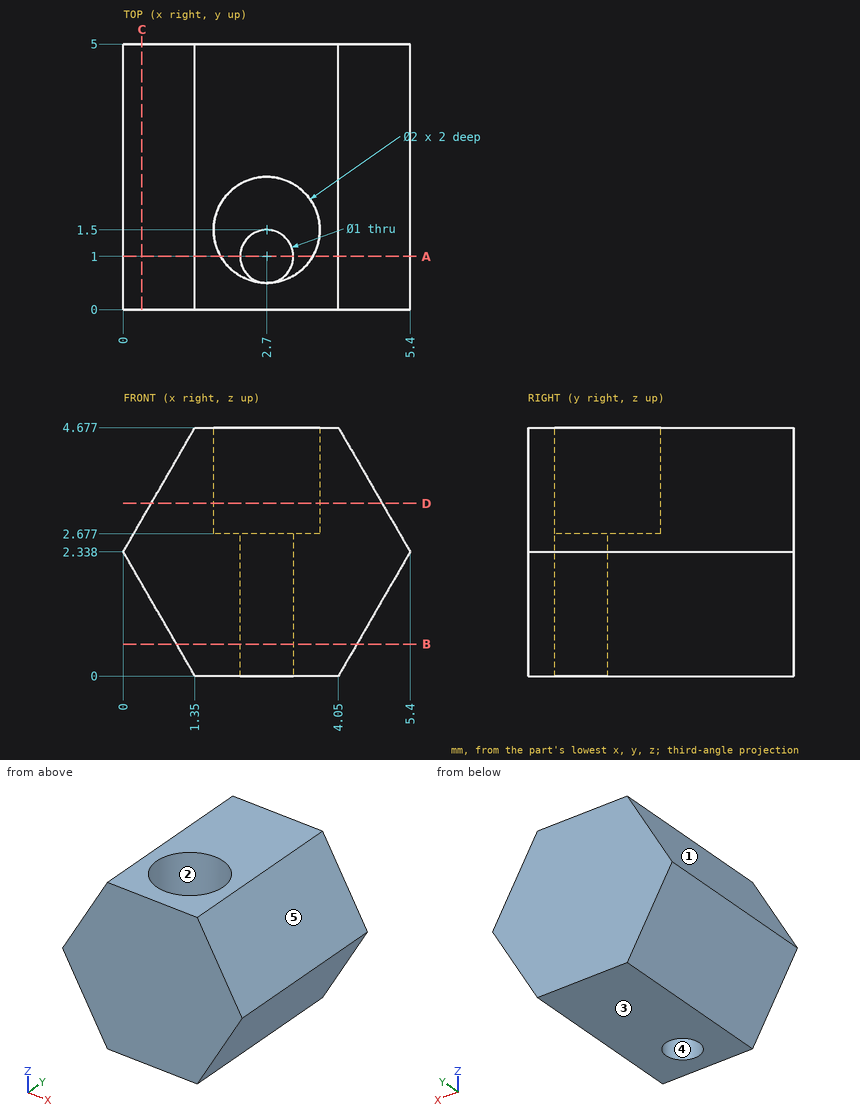
Geometry check sheet. Reference: drawing and pictorial views, mm from the part's lowest x, y, z. A direction names the side the tool comes from. Give positions to 0.01 mm unless a question says otherwise; leave off trailing zeros. Loops run counter-clockwise (first coordinate to the right, second up) from the corner with the lowest first, then second, coordinate; pieces in that order, holes last. Notation, with made-up numbers: M 15,33 L 20,33 A23 ccw 20,49 Z; hole C 69,47.25 d8. An arc over 180 degrees is marked long. Use a Markdown table: item, result. Add a question column.
Q1. Scan lines: line 1 along Y through (x, z) = (2.7, 2.05); line 2 along Y through (x, z) = (2.7, 3.25); line 3 along X through (y, z) = (1, 1.7). Record each from-to range of solid material in increasing order. Write a range as [from, to].
Q2. Go/stop test with flat-tipped pins: pin 1 (1 mm diameter, centred on y = 3, z = 1, fed in from +X) (1 decimal); pin 2 (1 mm diameter, centred on x = 5, y = 2.5, fed in from -Z); pin 3 (1.6 mm diameter, centred on x = 2.7, y = 1.5, fed in from +Z). Record where each tip stops, or that it passes through.
Q3. Tool access check on the marked faces 1 and 2. Record the directions out of +Z, -Z, +X, -X, +Y, -Y that give a thin tool (end or side, any length) a straight path to the whole face; none if there is none.
Q4. Sectioned sample at B-B, the plane z = 0.6. Record the cut outline in (x, y).
Q5. Sectioned sample at C-C, the plane x = 0.35. Record the cut outline in (y, z) (1 decimal).
Q6. Mould release check, pull along X, two halves, no side actions. Record for the marked faces 3, 4 and 5: pulls with the +X half, pulls with the -X half, needs draft (parallel to the pull), parting line crosses it, or undercut.
Q7. Sectioned sample at D-D, the plane z = 3.25. Record the cut outline in (x, y).
Q8. Sectioned sample at A-A, the plane y = 1. Record the cut outline in (x, z).
Verdict:
| question | item | result |
|---|---|---|
| 1 | line 1 | [0, 0.5], [1.5, 5] |
| 1 | line 2 | [0, 0.5], [2.5, 5] |
| 1 | line 3 | [0.37, 2.2], [3.2, 5.03] |
| 2 | pin 1 | x = 4.9 |
| 2 | pin 2 | z = 0.78 |
| 2 | pin 3 | z = 2.68 |
| 3 | face 1 | +Z, -X, +Y, -Y |
| 3 | face 2 | +Z |
| 4 | outline | M 1,0 L 4.4,0 L 4.4,5 L 1,5 Z; hole C 2.7,1 d1 |
| 5 | outline | M 0,1.7 L 5,1.7 L 5,2.9 L 0,2.9 Z |
| 6 | face 3 | needs draft |
| 6 | face 4 | undercut |
| 6 | face 5 | pulls with the +X half |
| 7 | outline | M 0.53,0 L 4.87,0 L 4.87,5 L 0.53,5 Z; hole C 2.7,1.5 d2 |
| 8 | outline | M 0,2.34 L 1.35,0 L 2.2,0 L 2.2,2.68 L 1.83,2.68 L 1.83,4.68 L 1.35,4.68 Z; M 3.2,0 L 4.05,0 L 5.4,2.34 L 4.05,4.68 L 3.57,4.68 L 3.57,2.68 L 3.2,2.68 Z |
